Here's how the part is built. I have some questions about the finished solid (model axes, mm). A direction names the side the tool comes from. Coordinates: 2 decimals unless noted, no trailing zeros. Write each loop counter-clockwise with the first axis right and the second up, starting at its lowest first coordinate (ties: lowest second). Pieces come first, ordered by that corner, then holes.
Item 1: I want a section at C-C (x = 4.5). Please give me the cut outline in (y, z), and give its area (3 significant figures).
Item 2: I want a section at B-B (z = 6.5). Please give me the cut outline in (x, y), and give its area (3 significant figures).
Item 3: For faces 1 (the face through (3, 15, 3.5)), 2 (the face through (0, -11, 11)), which set-ups out of +Z, -Z, +X, -X, +Y, -Y let a thin tool reach every point of the face, with its end or its side?
Item 4: I'm going to push flat-ended pins straight in: P1, Ø1.3, axis at y = 13.5, z = 0, coming from the -X side; P2, Ø12, axis at y = -4.5, z = 2.5, coming from the -X side; P3, Ø10, axis at y = -7.5, z = -2, coming from the +X side; P4, Ø1, axis at x = 16.5, z = 8, coming from the -Y side. Where does each tip first touch, or does it pass through?
Item 5: Please list where these lines run through material, in increasing order: line 1 (X direction, y = -0.1, z = 0); line 2 (Y direction, x = 4.25, z = 9); line 3 (Z direction, x = 7.5, y = -4).
Item 6: I want a section at A-A (x = 13.25). Please give me the cut outline in (y, z), and give its area (3 significant figures).
Item 7: If we mould it in two halves opening along Z, with no side actions, what happens to faces 3 (the face through (18, 0, -2)), 4 (the face through (16.5, 0.01, 0.46)), 5 (the face through (16.3, -1, 0.6))? For each: pulls with the +Z half, pulls with the -Z half, needs draft (parallel to the pull), parting line crosses it, or undercut.
from build123d import *

# Parameters (mm, degrees)
REVOLVE_2_ANGLE     = 180
SKETCH_2_W          = 5
SKETCH_2_H          = 2
EXTRUDE_1_DEPTH     = 4
SKETCH_3_R          = 1
CUT_EXTRUDE_1_DEPTH = 5
FILLET_1_R          = 2.5
FILLET_2_R          = 2.5
SKETCH_4_W          = 6.7
SKETCH_4_H          = 7
CUT_EXTRUDE_2_DEPTH = 15


with BuildPart() as part:
    # 草图1 → 旋转2 (revolve)
    with BuildSketch(Plane(origin=(0, 0, 0), x_dir=(0, 0, -1), z_dir=(1, 0, 0))):
        with BuildLine():
            Line((-16, 0), (-15, 0))
            ThreePointArc((-15, 0), (0, 15), (15, 0))
            Line((15, 0), (16, 0))
            ThreePointArc((16, 0), (0, 16), (-16, 0))
        make_face()
    revolve(axis=Axis((0, 0, -15), (0, 0, -1)), revolution_arc=REVOLVE_2_ANGLE)

    # 草图2 → 凸台-拉伸1 (add)
    with BuildSketch(Plane(origin=(15, 0, 0), x_dir=(0, 0, -1), z_dir=(1, 0, 0))):
        Rectangle(SKETCH_2_W, SKETCH_2_H)
    extrude(amount=EXTRUDE_1_DEPTH)

    # 草图3 → 切除-拉伸1 (cut)
    with BuildSketch(Plane(origin=(0, 1, 0), x_dir=(1, 0, 0), z_dir=(0, 1, 0))):
        with Locations(Location((17.385905148, 0, 0), (0, 0, 270))):
            Circle(SKETCH_3_R)
    extrude(amount=-CUT_EXTRUDE_1_DEPTH, mode=Mode.SUBTRACT)

    # 圆角1
    fillet_1_edges = [part.edges().sort_by_distance(p)[0] for p in [
        (19, 0, -2.5),
    ]]
    fillet(fillet_1_edges, radius=FILLET_1_R)

    # 圆角2
    fillet_2_edges = [part.edges().sort_by_distance(p)[0] for p in [
        (19, 0, 2.5),
    ]]
    fillet(fillet_2_edges, radius=FILLET_2_R - 0.0001)  # a hair under: the kernel refuses the full size

    # 草图4 → 切除-拉伸2 (cut)
    with BuildSketch(Plane(origin=(0, 18.626931023, 0), x_dir=(1, 0, 0), z_dir=(0, 1, 0))):
        with Locations((3.35, 0)):
            Rectangle(SKETCH_4_W, SKETCH_4_H)
    extrude(amount=-CUT_EXTRUDE_2_DEPTH, mode=Mode.SUBTRACT)


solid = part.part
Answer:
1. outline: (13.87, -3.5) arc R14.31 cw (long way) to (13.87, 3.5) - (14.95, 3.5) arc R15.35 ccw (long way) to (14.95, -3.5) - close
1. area: 90.0 mm2
2. outline: (0, -14.62) arc R14.62 ccw to (0, 14.62) - (0, 13.52) arc R13.52 cw to (0, -13.52) - close
2. area: 48.7 mm2
3. face 1: -X, +Y
3. face 2: +Z, -Z, -X, +Y, -Y
4. P1: stops at x = 6.7
4. P2: stops at x = 10.04
4. P3: stops at x = 15.76
4. P4: passes through
5. line 1: x = 15 to 16.39, 18.39 to 19
5. line 2: y = -12.53 to -11.22, 11.22 to 12.53
5. line 3: z = -13.56 to -12.36, 12.36 to 13.56
6. outline: circle Ø17.94 at (0, 0); hole circle Ø14.06 at (0, 0)
6. area: 97.4 mm2
7. face 3: pulls with the -Z half
7. face 4: undercut
7. face 5: needs draft
